from build123d import *

# Parameters (mm, degrees)
SKIZZE1_W                            = 32.76
SKIZZE1_H                            = 1.995
FASE1_SIZE                           = 0.2
SCHNITT_LINEAR_AUSTRAGEN1_DEPTH      = 33.881265943
SCHNITT_LINEAR_AUSTRAGEN1_DEPTH_BACK = 33.881265943


with BuildPart() as part:
    # Skizze1 → Rotation1 (revolve)
    with BuildSketch(Plane(origin=(0, 0, 0), x_dir=(0, 0, -1), z_dir=(1, 0, 0)), mode=Mode.PRIVATE) as rotation1_sk:
        with Locations((16.38, 0.9975)):
            Rectangle(SKIZZE1_W, SKIZZE1_H)
    revolve(rotation1_sk.sketch.rotate(Axis((0, 0, 50.516901408), (0, 0, -1)), 90), axis=Axis((0, 0, 50.516901408), (0, 0, -1)))

    # Fase1
    fase1_edges = [part.edges().sort_by_distance(p)[0] for p in [
        (-1.995, 0, -32.76),
        (-1.995, 0, 0),
    ]]
    chamfer(fase1_edges, length=FASE1_SIZE)

    # Skizze2 → Schnitt-Linear austragen1 (cut, two sides: drawn at the far end of the back side and taken through both)
    with BuildSketch(Plane(origin=(0, 0, 0), x_dir=(1, 0, 0), z_dir=(0, 1, 0)).offset(-SCHNITT_LINEAR_AUSTRAGEN1_DEPTH_BACK)):
        with BuildLine():
            Line((-6.2, 26.76), (-1.8, 26.76))
            ThreePointArc((-1.8, 26.76), (-1.729289322, 26.789289322), (-1.7, 26.86))
            Line((-1.7, 26.86), (-1.7, 31.16))
            ThreePointArc((-1.7, 31.16), (-1.729289322, 31.230710678), (-1.8, 31.26))
            Line((-1.8, 31.26), (-6.2, 31.26))
            Line((-6.2, 31.26), (-6.2, 26.76))
        make_face()
        with BuildLine():
            Line((1.7, 26.86), (1.7, 31.16))
            ThreePointArc((1.7, 31.16), (1.729289322, 31.230710678), (1.8, 31.26))
            Line((1.8, 31.26), (6.2, 31.26))
            Line((6.2, 31.26), (6.2, 26.76))
            Line((6.2, 26.76), (1.8, 26.76))
            ThreePointArc((1.8, 26.76), (1.729289322, 26.789289322), (1.7, 26.86))
        make_face()
    extrude(amount=SCHNITT_LINEAR_AUSTRAGEN1_DEPTH + SCHNITT_LINEAR_AUSTRAGEN1_DEPTH_BACK, mode=Mode.SUBTRACT)


solid = part.part
The model under review builds one solid part; all positions refer to its coordinate system, in mm. A direction names the side the tool comes from. Coordinates: 2 decimals unless noted, no trailing zeros. Loops run counter-clockwise (first coordinate to the right, second up) from the corner with the lowest first, then second, coordinate; pieces in that order, holes last. Notation, with made-up numbers: (32, 82) -> (86, 82) arc R32 ccw to (86, 119) -> close; hole circle Ø6 at (20.25, 73.25). An arc over 180 degrees is marked (long way). Use a Markdown table: item, result. Add a question column.
1. Clearance check with flat-ended pins moving along their axes: pin 1 Ø2 at (y, z) = (0, -29) entering from +X; pin 2 Ø1 at (y, z) = (-0.5, -28) entering from -X. State where each tip first meets the part, or that it passes through.
2. To check wall thickness, follow line 1 (Y direction, x = -1.8, z = -14); line 2 (X direction, y = -0.85, z = -11). State the ranges of each line that lie inside material, in increasing order.
3. Add section A-A on y = 0. Write out the cut boundary in (x, z) (3 decimals), plus the area to 3 significant figures.
4. Add section C-C on z = -11.5. Write out the cut boundary in (x, y) (3 decimals).
5. Draft analysis for pull direction Z (two halves, no side actions). For faces 1 (the face through (0, 0, 0)), 2 (the face through (-1.7, 0, -29)), 3 (the face through (0, 0, -32.76)), state which applies: pulls with the +Z half, pulls with the -Z half, needs draft (parallel to the pull), parting line crosses it, or undercut.
6. Machinability: for faces 4 (the face through (-1.993, -0.088, -16.607)), 5 (the face through (1.7, 0, -29)), which of the approach directions +Z, -Z, +X, -X, +Y, -Y give a long, thin tool a straight path to every point of the face, cutting with its end or side? Answer none if there is none.
7. Add section B-B on z = -27.5. Write out the cut boundary in (x, y) (3 decimals).
Returned:
| question | item | result |
|---|---|---|
| 1 | pin 1 | stops at x = 1.7 |
| 1 | pin 2 | stops at x = -1.7 |
| 2 | line 1 | y = -0.86 to 0.86 |
| 2 | line 2 | x = -1.8 to 1.8 |
| 3 | outline | (-1.995, -32.56) -> (-1.795, -32.76) -> (1.795, -32.76) -> (1.995, -32.56) -> (1.995, -31.26) -> (1.8, -31.26) arc R0.1 cw to (1.7, -31.16) -> (1.7, -26.86) arc R0.1 cw to (1.8, -26.76) -> (1.995, -26.76) -> (1.995, -0.2) -> (1.795, 0) -> (-1.795, 0) -> (-1.995, -0.2) -> (-1.995, -26.76) -> (-1.8, -26.76) arc R0.1 cw to (-1.7, -26.86) -> (-1.7, -31.16) arc R0.1 cw to (-1.8, -31.26) -> (-1.995, -31.26) -> close |
| 3 | area | 128 mm² |
| 4 | outline | circle Ø3.99 at (0, 0) |
| 5 | face 1 | pulls with the +Z half |
| 5 | face 2 | undercut |
| 5 | face 3 | pulls with the -Z half |
| 6 | face 4 | +Z, -Z |
| 6 | face 5 | +X, +Y, -Y |
| 7 | outline | (-1.7, -1.044) arc R1.995 ccw to (1.7, -1.044) -> (1.7, 1.044) arc R1.995 ccw to (-1.7, 1.044) -> close |
